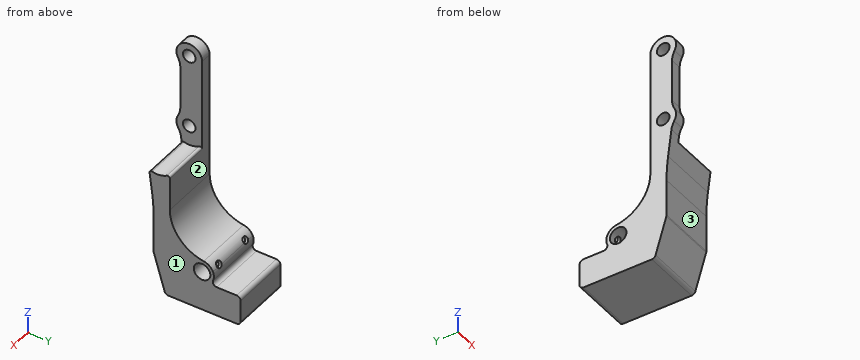
from build123d import *
from build123d.topology import SkipClean

# Parameters (mm, degrees)
SKETCH_1_R               = 4.2
SKETCH_1_R_2             = 3.2
EXTRUDE_1_DEPTH          = 30
CUT_EXTRUDE_1_DEPTH      = 125.586877319
CUT_EXTRUDE_1_DEPTH_BACK = 125.586877319
SKETCH_2_R               = 5
SKETCH_4_R               = 8
CUT_EXTRUDE_3_DEPTH      = 24.3
CUT_EXTRUDE_4_DEPTH      = 24.3
CUT_EXTRUDE_5_REACH      = 105.181
CUT_EXTRUDE_5_END_RADIUS = 4.2
SKETCH_7_R               = 1.7
FILLET_1_R               = 2
FILLET_2_R               = 100
FILLET_4_R               = 2
FILLET_5_R               = 1
FILLET_6_R               = 10


with BuildPart() as part:
    # ｽｹｯﾁ1 → ﾎﾞｽ - 押し出し1 (new body)
    with BuildSketch(Plane(origin=(0, 0, 0), x_dir=(0, 0, -1), z_dir=(1, 0, 0))):
        with BuildLine():
            Line((0, 0), (0, -38))
            Line((0, -38), (-20, -44))
            Line((-20, -44), (-45, -44))
            Line((-45, -44), (-67.30958424, -46.8))
            ThreePointArc((-67.30958424, -46.8), (-72, -48.8), (-76.69041576, -46.8))
            Line((-76.69041576, -46.8), (-104.30958424, -46.8))
            ThreePointArc((-104.30958424, -46.8), (-114.979130372, -44.849509757), (-109, -35.8))
            Line((-109, -35.8), (-73.332546795, -35.8))
            Line((-73.332546795, -35.8), (-72, -35.8))
            Line((-72, -35.8), (-45.735384202, -35.8))
            ThreePointArc((-45.735384202, -35.8), (-32.638114962, -30.91494421), (-25.938934816, -18.646153846))
            ThreePointArc((-25.938934816, -18.646153846), (-24.759789788, -15.847001072), (-22.360864108, -13.983994139))
            ThreePointArc((-22.360864108, -13.983994139), (-18.282275098, -13.751137403), (-15, -16.18337521))
            Line((-15, -16.18337521), (-15, 0))
            Line((-15, 0), (0, 0))
        make_face()
        with Locations((-20, -19.5)):
            Circle(SKETCH_1_R, mode=Mode.SUBTRACT)
        with Locations((-109, -42.3)):
            Circle(SKETCH_1_R_2, mode=Mode.SUBTRACT)
        with Locations((-72, -42.3)):
            Circle(SKETCH_1_R_2, mode=Mode.SUBTRACT)
    extrude(amount=EXTRUDE_1_DEPTH)

    # ｽｹｯﾁ2 → ｶｯﾄ - 押し出し1 (cut, two sides: drawn at the far end of the back side and taken through both)
    with BuildSketch(Plane(origin=(0, -35.8, 0), x_dir=(1, 0, 0), z_dir=(0, 1, 0)).offset(-CUT_EXTRUDE_1_DEPTH_BACK)):
        with Locations(Location((15, -83.6, 0), (0, 0, 270))):
            Circle(SKETCH_2_R)
    extrude(amount=CUT_EXTRUDE_1_DEPTH + CUT_EXTRUDE_1_DEPTH_BACK, mode=Mode.SUBTRACT)

    # ｽｹｯﾁ4 → ｶｯﾄ - 押し出し3 (cut)
    with BuildSketch(Plane(origin=(30, 0, 0), x_dir=(0, 0, -1), z_dir=(1, 0, 0))):
        with Locations((-72, -42.3)):
            Circle(SKETCH_4_R)
        with Locations((-109, -42.3)):
            Circle(SKETCH_4_R)
    extrude(amount=-CUT_EXTRUDE_3_DEPTH, mode=Mode.SUBTRACT)

    # ｽｹｯﾁ5 → ｶｯﾄ - 押し出し4 (cut)
    with BuildSketch(Plane(origin=(30, 0, 0), x_dir=(0, 0, -1), z_dir=(1, 0, 0))):
        with BuildLine():
            Line((-109, -32.3), (-72, -32.3))
            ThreePointArc((-72, -32.3), (-62, -42.3), (-72, -52.3))
            Line((-72, -52.3), (-109, -52.3))
            ThreePointArc((-109, -52.3), (-119, -42.3), (-109, -32.3))
        make_face()
    extrude(amount=-CUT_EXTRUDE_4_DEPTH, mode=Mode.SUBTRACT)

    # ｶｯﾄ - 押し出し5: up to this cylinder (the profile starts outside it)
    with SkipClean():  # the faces are left unmerged after this step: merging them gives an invalid solid
        cut_extrude_5_end = Plane(origin=(15, -19.5, 20), z_dir=(-1, 0, 0)) * Cylinder(CUT_EXTRUDE_5_END_RADIUS, 239.762, mode=Mode.PRIVATE)
        # ｽｹｯﾁ7 → ｶｯﾄ - 押し出し5 (cut, up to the surface)
        with BuildSketch(Plane(origin=(30, -14.303847577, 23), x_dir=(1, 0, 0), z_dir=(0, 0.866025403784436, 0.5000000000000043)), mode=Mode.PRIVATE) as cut_extrude_5_sk1:
            with Locations(Location((-5, 0, 0), (0, 0, 270))):
                Circle(SKETCH_7_R)
        cut_extrude_5_tool1 = extrude(cut_extrude_5_sk1.sketch, amount=-CUT_EXTRUDE_5_REACH, mode=Mode.PRIVATE) - cut_extrude_5_end
        add(cut_extrude_5_tool1.solids().sort_by_distance((25, -14.303848, 23))[0], mode=Mode.SUBTRACT)
        # ｽｹｯﾁ7 → ｶｯﾄ - 押し出し5 (cut, up to the surface)
        with BuildSketch(Plane(origin=(30, -14.303847577, 23), x_dir=(1, 0, 0), z_dir=(0, 0.866025403784436, 0.5000000000000043)), mode=Mode.PRIVATE) as cut_extrude_5_sk2:
            with Locations(Location((-25, 0, 0), (0, 0, 270))):
                Circle(SKETCH_7_R)
        cut_extrude_5_tool2 = extrude(cut_extrude_5_sk2.sketch, amount=-CUT_EXTRUDE_5_REACH, mode=Mode.PRIVATE) - cut_extrude_5_end
        add(cut_extrude_5_tool2.solids().sort_by_distance((5, -14.303848, 23))[0], mode=Mode.SUBTRACT)

    # ﾌｨﾚｯﾄ1
    fillet_1_edges = [part.edges().sort_by_distance(p)[0] for p in [
        (15, -16.18337521, 15),
    ]]
    fillet(fillet_1_edges, radius=FILLET_1_R)

    # ﾌｨﾚｯﾄ2
    fillet_2_edges = [part.edges().sort_by_distance(p)[0] for p in [
        (15, -44, 45),
    ]]
    fillet(fillet_2_edges, radius=FILLET_2_R)

    # ﾌｨﾚｯﾄ4
    fillet_4_edges = [part.edges().sort_by_distance(p)[0] for p in [
        (15, 0, 0),
        (15, -38, 0),
        (15, -44, 20),
        (15, 0, 15),
    ]]
    fillet(fillet_4_edges, radius=FILLET_4_R)

    # ﾌｨﾚｯﾄ5
    fillet_5_edges = [part.edges().sort_by_distance(p)[0] for p in [
        (17.85, -46.23485742, 62.80669281),
        (17.85, -35.8, 64.400657923),
    ]]
    fillet(fillet_5_edges, radius=FILLET_5_R)

    # ﾌｨﾚｯﾄ6
    fillet_6_edges = [part.edges().sort_by_distance(p)[0] for p in [
        (2.85, -46.8, 67.30958424),
        (2.85, -46.8, 76.69041576),
        (2.85, -46.8, 104.30958424),
    ]]
    fillet(fillet_6_edges, radius=FILLET_6_R)


solid = part.part
CAD build for the part. Positions are in the model's coordinates, mm. Face numbers are marked on the shaded views. A direction names the side the tool comes from. Coordinates: 2 decimals unless noted, no trailing zeros. Write each loop counter-clockwise with the first axis right and the second up, starting at its lowest first coordinate (ties: lowest second). Pieces come first, ordered by that corner, then holes. Notation, with made-up numbers: (-23.75, -20.5) - (9.25, -20.5) arc R9 ccw to (9.25, -9.5) - close; hole circle Ø11 at (-8.5, 63). An arc over 180 degrees is marked (long way). Use a Markdown table: item, result. Add a question column.
Item 1: Band-saw the part on D-D, the plane x = 9.5. Give the cut face in (y, z), and give its area (3 significant figures).
Item 2: Drill centre lines: L1, parallel to Y at x = 4.5, z = 72; L2, parallel to Z at x = 23, y = -10; L3, parallel to Y at x = 23, z = 20. Where is each one in solid material? Low to high. Write a range as from..to.
Item 3: Band-saw the part on A-A, the plane y = -42.3. Give the cut face in (x, z).
Item 4: 3-axis set-ups, long thin cutter, end or side, ignore diameter. For the marked faces 1, 2 and 3: which of +Z, -Z, +X, -X, +Y, -Y reach the whole face in a straight line?
Item 5: Flat gauge pins, fed straight in: pin 1 (12 mm diameter, centred on y = -42, z = 79.5, fed in from +X); pin 2 (1.5 mm diameter, centred on x = 22, z = 56.5, fed in from -Y); pin 3 (9 mm diameter, centred on x = 16.5, z = 30, fed in from -Y). Where does each tip first touch, or does it go through?
Item 6: Band-saw the part on C-C, the plane y = -22. Give the cut face in (x, z).
Item 7: Band-saw the part on B-B, the plane z = 72. Give the cut face in (x, y), and give its area (3 significant figures).
Numbers:
| question | item | result |
|---|---|---|
| 1 | outline | (-46.04, 61.22) - (-44.78, 51.2) arc R100 cw to (-44, 38.75) - (-44, 20.29) arc R2 ccw to (-43.92, 19.72) - (-38.43, 1.43) arc R2 ccw to (-36.51, 0) - (-2, 0) arc R2 ccw to (0, 2) - (0, 13) arc R2 ccw to (-2, 15) - (-12.08, 15) arc R2 cw to (-13.94, 17.75) arc R6 ccw to (-18.65, 25.94) arc R20 cw to (-35.8, 45.74) - (-35.8, 62.47) arc R1 ccw to (-37.3, 63.34) arc R10 cw to (-44.79, 62.32) arc R1 ccw to start; hole circle Ø8.4 at (-19.5, 20) |
| 1 | area | 1,270 mm2 |
| 2 | L1 | -48.8..-45.5, -39.1..-35.8 |
| 2 | L2 | 0..15 |
| 2 | L3 | -43.98..-23.7, -15.3..-13.5 |
| 3 | outline | (0, 14.33) - (30, 14.33) - (30, 62) - (5.7, 62) - (5.7, 68.8) - (0, 68.8) - close; (0, 75.2) - (5.7, 75.2) - (5.7, 105.8) - (0, 105.8) - close; (0, 112.2) - (5.7, 112.2) - (5.7, 115.5) - (0, 115.5) - close |
| 4 | face 1 | +Z, -Z, +X, +Y, -Y |
| 4 | face 2 | +Z, +X, -X, +Y |
| 4 | face 3 | -Z, +X, -X, -Y |
| 5 | pin 1 | x = 5.7 |
| 5 | pin 2 | y = -45.54 |
| 5 | pin 3 | y = -44 |
| 6 | outline | (0, 0) - (30, 0) - (30, 16.63) - (0, 16.63) - close; (0, 23.37) - (30, 23.37) - (30, 26.72) - (0, 26.72) - close |
| 7 | outline | (0, -48.8) - (5.7, -48.8) - (5.7, -45.5) - (0, -45.5) - close; (0, -39.1) - (5.7, -39.1) - (5.7, -35.8) - (0, -35.8) - close |
| 7 | area | 37.6 mm2 |
